Autodesk Inventor part; units mm, degrees
ref_plane "Work Plane1" through (0, 51.5, 0) normal (0, 1, 0) x (1, 0, 0)
ref_plane "YZ Plane" through (0, 0, 0) normal (1, 0, 0) x (0, 1, 0)
ref_plane "XZ Plane" through (0, 0, 0) normal (0, 1, 0) x (-1, 0, 0)
sketch "Sketch1" plane through (0, 0, 0) normal (0, 1, 0) x (-1, 0, 0)
  circle A0 centre (0, 0) radius 17.5
  dimension "d0" = 35
extrude "Extrusion1" add sketch "Sketch1" along normal blind 103
sketch "Sketch2" plane through (0, 103, 0) normal (0, 1, 0) x (1, 0, 0)
  circle A0 centre (0, 0) radius 3
  circle A1 centre (0, 0) radius 9
  circle A2 centre (0, 0) radius 17.5
  dimension "d3" = 6
  dimension "d4" = 18
extrude "Extrusion2" cut sketch "Sketch2" against normal blind 2 contours A2
extrude "Extrusion3" cut sketch "Sketch2" against normal through all contours A0
ref_plane "Work Plane1" through (0, 51.5, 0) normal (0, 1, 0) x (1, 0, 0)
mirror "Mirror1" about plane through (0, 51.5, 0) normal (0, 1, 0) of "Extrusion2"
properties part number "roller"
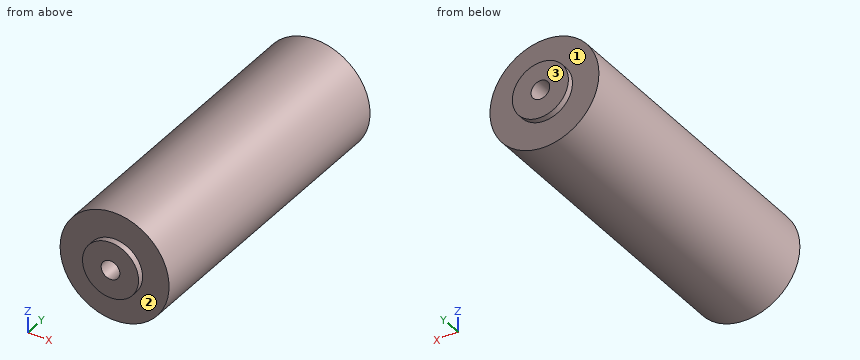
Check sheet for the modelled part. Datum: model origin and axes. Units: mm. Face numbers are marked on the shaded views. A direction names the side the tool comes from. Coordinates: 2 decimals unless noted, no trailing zeros. Order: outer loops, then holes, each group sorted by start corner. A loop starts at its lowest first (then second) coordinate and runs counter-clockwise, first axis right, second up. Notation, with made-up numbers: (-32, -24.75) -> (-24, -24.75) arc R16 cw to (-24, -11.75) -> close; hole circle Ø5 at (-13.5, 68). An arc over 180 degrees is marked (long way). Write item = value, one per line. Start each with the question number.
1) Access from +Z, -Z, +X, -X, +Y, -Y to the whole of each face (thin tool, end or side, straight path). Record for the marked faces 1, 2 and 3.
2) Cross-section at C-C (y = 13). Enter the section's corners in (x, z), then the cut area to 3 significant figures.
3) Cross-section at D-D (z = 14). Enter the section's corners in (x, y), then the cut area to 3 significant figures.
4) Cross-section at A-A (z = 0). Enter the section's corners in (x, y), then the cut area to 3 significant figures.
5) Go/stop test with flat-tipped pins: P1, Ø1.5, axis at x = 5, z = 10, coming from the +Y side; P2, Ø5, axis at y = 42.5, z = -13.5, coming from the -X side; P3, Ø1.5, axis at x = -6, y = 68.5, coming from the +Z side. Record where each tip stops, or that it passes through.
6) Material ranges on L1, parallel to Z at x = 0, y = 39.5; L2, parallel to Y at x = -4.5, z = 11, recorded low to high.
7) Cross-section at B-B (x = 0). Enter the section's corners in (y, z).
Ans:
q1.face_1 = +Y
q1.face_2 = -Y
q1.face_3 = +Z, -Z, +X, -X, +Y
q2.outline = circle Ø35 at (0, 0); hole circle Ø6 at (0, 0)
q2.area = 934 mm²
q3.outline = (-10.5, 2) -> (10.5, 2) -> (10.5, 101) -> (-10.5, 101) -> close
q3.area = 2,080 mm²
q4.outline = (-17.5, 2) -> (-9, 2) -> (-9, 0) -> (-3, 0) -> (-3, 103) -> (-9, 103) -> (-9, 101) -> (-17.5, 101) -> close; (3, 0) -> (9, 0) -> (9, 2) -> (17.5, 2) -> (17.5, 101) -> (9, 101) -> (9, 103) -> (3, 103) -> close
q4.area = 2,920 mm²
q5.P1 = 101
q5.P2 = -13.61
q5.P3 = 16.69
q6.L1 = -17.5 to -3, 3 to 17.5
q6.L2 = 2 to 101
q7.outline = (0, -9) -> (2, -9) -> (2, -17.5) -> (101, -17.5) -> (101, -9) -> (103, -9) -> (103, -3) -> (0, -3) -> close; (0, 3) -> (103, 3) -> (103, 9) -> (101, 9) -> (101, 17.5) -> (2, 17.5) -> (2, 9) -> (0, 9) -> close
